```python
from build123d import *

# Parameters (mm, degrees)
SKIZZE1_R                       = 90
AUFSATZ_LINEAR_AUSTRAGEN1_DEPTH = 5
SKIZZE2_W                       = 6
SKIZZE2_H                       = 10
AUFSATZ_LINEAR_AUSTRAGEN2_DEPTH = 14
FASE1_SIZE                      = 14
SKIZZE3_R                       = 2.15
SCHNITT_LINEAR_AUSTRAGEN1_DEPTH = 42
KREISMUSTER1_COUNT              = 3
FASE1_OF_KREISMUSTER1_SIZE      = 14
AUFSATZ_LINEAR_AUSTRAGEN3_DEPTH = 3
AUFSATZ_LINEAR_AUSTRAGEN4_DEPTH = 3
SCHNITT_LINEAR_AUSTRAGEN2_REACH = 129.754
SKIZZE7_R                       = 1.75
KREISMUSTER2_COUNT              = 4
SCHNITT_LINEAR_AUSTRAGEN3_REACH = 130.69
SKIZZE8_R                       = 10
FASE2_SIZE                      = 0.5


with BuildPart() as part:
    # Skizze1 → Aufsatz-Linear austragen1 (new body)
    with BuildSketch(Plane(origin=(0, 0, 0), x_dir=(1, 0, 0), z_dir=(0, 1, 0))):
        with Locations(Location((0, 0, 0), (0, 0, 270))):
            Circle(SKIZZE1_R)
    extrude(amount=AUFSATZ_LINEAR_AUSTRAGEN1_DEPTH)

    # Skizze2 → Aufsatz-Linear austragen2 (add)
    with BuildSketch(Plane.XZ):
        with Locations((-18, 35)):
            Rectangle(SKIZZE2_W, SKIZZE2_H)
        with Locations((18, 35)):
            Rectangle(SKIZZE2_W, SKIZZE2_H)
    aufsatz_linear_austragen2 = extrude(amount=AUFSATZ_LINEAR_AUSTRAGEN2_DEPTH)

    # Fase1
    fase1_edges = [part.edges().sort_by_distance(p)[0] for p in [
        (18, 0, 40),
        (-18, 0, 40),
    ]]
    chamfer(fase1_edges, length=FASE1_SIZE - 0.0001)  # a hair under: the kernel refuses the full size

    # Skizze3 → Schnitt-Linear austragen1 (cut)
    with BuildSketch(Plane(origin=(21, 0, 0), x_dir=(0, 0, -1), z_dir=(1, 0, 0))):
        with Locations((-35, -7)):
            Circle(SKIZZE3_R)
    schnitt_linear_austragen1 = extrude(amount=-SCHNITT_LINEAR_AUSTRAGEN1_DEPTH, mode=Mode.SUBTRACT)

    # Kreismuster1: Aufsatz-Linear austragen2, Schnitt-Linear austragen1 ×3 about axis
    kreismuster1_axis = Axis((0, 0, 0), (0, 1, 0))
    add([aufsatz_linear_austragen2.rotate(kreismuster1_axis, i * 360 / KREISMUSTER1_COUNT) for i in range(1, KREISMUSTER1_COUNT)])
    add([schnitt_linear_austragen1.rotate(kreismuster1_axis, i * 360 / KREISMUSTER1_COUNT) for i in range(1, KREISMUSTER1_COUNT)], mode=Mode.SUBTRACT)

    # Fase1 of Kreismuster1
    fase1_of_kreismuster1_edges = [part.edges().sort_by_distance(p)[0] for p in [
        (25.641016151, 0, -35.588457268),
        (43.641016151, 0, -4.411542732),
        (-43.641016151, 0, -4.411542732),
        (-25.641016151, 0, -35.588457268),
    ]]
    chamfer(fase1_of_kreismuster1_edges, length=FASE1_OF_KREISMUSTER1_SIZE - 0.0001)  # a hair under: the kernel refuses the full size

    # Skizze4 → Aufsatz-Linear austragen3 (add)
    with BuildSketch(Plane.XZ):
        with BuildLine():
            ThreePointArc((-70.255477849, -23.241510972), (-64.08587988, 37), (-15, 72.463784058))
            Line((-15, 72.463784058), (-15, 78.581168228))
            ThreePointArc((-15, 78.581168228), (-69.282032303, 40), (-75.553287944, -26.300203057))
            Line((-75.553287944, -26.300203057), (-70.255477849, -23.241510972))
        make_face()
        with BuildLine():
            Line((15, 78.581168228), (15, 72.463784058))
            ThreePointArc((15, 72.463784058), (57.384666942, 46.722585545), (74, 0))
            ThreePointArc((74, 0), (73.057872132, -11.770612542), (70.255477849, -23.241510972))
            Line((70.255477849, -23.241510972), (75.553287944, -26.300203057))
            ThreePointArc((75.553287944, -26.300203057), (78.880488828, -13.336734317), (80, 0))
            ThreePointArc((80, 0), (61.64414003, 50.990195136), (15, 78.581168228))
        make_face()
        with BuildLine():
            ThreePointArc((55.255477849, -49.222273086), (0, -74), (-55.255477849, -49.222273086))
            Line((-55.255477849, -49.222273086), (-60.553287944, -52.280965171))
            ThreePointArc((-60.553287944, -52.280965171), (0, -80), (60.553287944, -52.280965171))
            Line((60.553287944, -52.280965171), (55.255477849, -49.222273086))
        make_face()
        with BuildLine():
            Line((15.480762114, -33.186533479), (18.480762114, -27.990381057))
            ThreePointArc((18.480762114, -27.990381057), (0, -33.541019662), (-18.480762114, -27.990381057))
            Line((-18.480762114, -27.990381057), (-15.480762114, -33.186533479))
            ThreePointArc((-15.480762114, -33.186533479), (0, -36.619666847), (15.480762114, -33.186533479))
        make_face()
        with BuildLine():
            ThreePointArc((-33.480762114, -2.009618943), (-29.047375097, 16.770509831), (-15, 30))
            Line((-15, 30), (-21, 30))
            ThreePointArc((-21, 30), (-31.713561768, 18.309833424), (-36.480762114, 3.186533479))
            Line((-36.480762114, 3.186533479), (-33.480762114, -2.009618943))
        make_face()
        with BuildLine():
            ThreePointArc((15, 30), (28.531695489, 17.633557569), (33.541019662, 0))
            ThreePointArc((33.541019662, 0), (33.525951891, -1.005261069), (33.480762114, -2.009618943))
            Line((33.480762114, -2.009618943), (36.480762114, 3.186533479))
            ThreePointArc((36.480762114, 3.186533479), (31.713561768, 18.309833424), (21, 30))
            Line((21, 30), (15, 30))
        make_face()
    extrude(amount=AUFSATZ_LINEAR_AUSTRAGEN3_DEPTH)

    # Skizze6 → Aufsatz-Linear austragen4 (add)
    with BuildSketch(Plane.XZ):
        with BuildLine():
            Line((-24.543328812, -76.142136894), (-25.319785948, -79.039914373))
            ThreePointArc((-25.319785948, -79.039914373), (-22.491358823, -83.938893859), (-17.592379337, -81.110466734))
            Line((-17.592379337, -81.110466734), (-16.815922202, -78.212689255))
            Line((-16.815922202, -78.212689255), (-24.543328812, -76.142136894))
        make_face()
        with BuildLine():
            Line((24.543328812, -76.142136894), (16.815922202, -78.212689255))
            Line((16.815922202, -78.212689255), (17.592379337, -81.110466734))
            ThreePointArc((17.592379337, -81.110466734), (22.491358823, -83.938893859), (25.319785948, -79.039914373))
            Line((25.319785948, -79.039914373), (24.543328812, -76.142136894))
        make_face()
    aufsatz_linear_austragen4 = extrude(amount=AUFSATZ_LINEAR_AUSTRAGEN4_DEPTH)

    # Skizze7 → Schnitt-Linear austragen2 (cut, up to next)
    with BuildSketch(Plane.XZ.offset(3), mode=Mode.PRIVATE) as schnitt_linear_austragen2_sk1:
        with Locations(Location((-21.456082643, -80.075190553, 0), (0, 0, 270))):
            Circle(SKIZZE7_R)
    schnitt_linear_austragen2_tool1 = extrude(schnitt_linear_austragen2_sk1.sketch, amount=-SCHNITT_LINEAR_AUSTRAGEN2_REACH, mode=Mode.PRIVATE) & part.part
    # Skizze7 → Schnitt-Linear austragen2 (cut, up to next)
    with BuildSketch(Plane.XZ.offset(3), mode=Mode.PRIVATE) as schnitt_linear_austragen2_sk2:
        with Locations(Location((21.456082643, -80.075190553, 0), (0, 0, 270))):
            Circle(SKIZZE7_R)
    schnitt_linear_austragen2_tool2 = extrude(schnitt_linear_austragen2_sk2.sketch, amount=-SCHNITT_LINEAR_AUSTRAGEN2_REACH, mode=Mode.PRIVATE) & part.part
    schnitt_linear_austragen2_1 = schnitt_linear_austragen2_tool1.solids().sort_by_distance((-21.456083, -3, -80.075191))[0]
    add(schnitt_linear_austragen2_1, mode=Mode.SUBTRACT)
    schnitt_linear_austragen2_2 = schnitt_linear_austragen2_tool2.solids().sort_by_distance((21.456083, -3, -80.075191))[0]
    add(schnitt_linear_austragen2_2, mode=Mode.SUBTRACT)
    schnitt_linear_austragen2 = schnitt_linear_austragen2_1 + schnitt_linear_austragen2_2  # Schnitt-Linear austragen2 as one shape, for the pattern or mirror that repeats it

    # Kreismuster2: Aufsatz-Linear austragen4, Schnitt-Linear austragen2 ×4 about axis
    kreismuster2_axis = Axis((0, 0, 0), (0, 1, 0))
    add([aufsatz_linear_austragen4.rotate(kreismuster2_axis, i * 360 / KREISMUSTER2_COUNT) for i in range(1, KREISMUSTER2_COUNT)])
    add([schnitt_linear_austragen2.rotate(kreismuster2_axis, i * 360 / KREISMUSTER2_COUNT) for i in range(1, KREISMUSTER2_COUNT)], mode=Mode.SUBTRACT)

    # Skizze8 → Schnitt-Linear austragen3 (cut, up to next)
    with BuildSketch(Plane(origin=(0, 5, 0), x_dir=(1, 0, 0), z_dir=(0, 1, 0)), mode=Mode.PRIVATE) as schnitt_linear_austragen3_sk1:
        with Locations(Location((0, 0, 0), (0, 0, 270))):
            Circle(SKIZZE8_R)
    schnitt_linear_austragen3_tool1 = extrude(schnitt_linear_austragen3_sk1.sketch, amount=-SCHNITT_LINEAR_AUSTRAGEN3_REACH, mode=Mode.PRIVATE) & part.part
    add(schnitt_linear_austragen3_tool1.solids().sort_by_distance((0, 5, 0))[0], mode=Mode.SUBTRACT)

    # Fase2
    fase2_edges = [part.edges().sort_by_distance(p)[0] for p in [
        (0, 5, -90),
    ]]
    chamfer(fase2_edges, length=FASE2_SIZE)


solid = part.part
```
Could you check a few things on this model? Use its own coordinates, in mm. A direction names the side the tool comes from. Round coordinates to 2 decimals unless told otherwise and drop trailing zeros. Loops run counter-clockwise (first coordinate to the right, second up) from the corner with the lowest first, then second, coordinate; pieces in that order, holes last.
Q1. For P1, Ø5.5, axis at x = 80.08, z = -21.46, coming from the -Y side; P2, Ø1.5, axis at y = -6, z = -11.5, coming from the +X side; P3, Ø11, axis at y = -9.5, z = 36.5, coming from the +X side, each with a flat end and sliding along its axis, tell me the tip position at first contact or that it passes through.
Q2. Thinking about a two-plate mould opening in Z: for faces 1 (the flat face through (0, -3, -76)), 2 (the flat face through (-44.418, -5.346, -1.396)), which applies, pulls with the +Z half, pulls with the -Z half, needs draft (parallel to the pull), parting line crosses it, or undercut?
Q3. I want a section at B-B (z = 35). Give the number of separate pieces and of enclosed holes in the cut face, and give its area (3 significant figures).
Q4. On a 3-axis mill with a long thin cutter (end or side, diameter ignored), from which of +Z, -Z, +X, -X, +Y, -Y can I reach the whole of each face in a straight line? I mean faces 3 (the flat face through (-15, -5, 39)), 4 (the flat face through (49.639, -7.098, -7.826)), 5 (the flat face through (18, -8, 30)), 6 (the flat face through (31.64, -7.1, -39)). Say none if no direction works.
Q5. I want a section at A-A (x = 0). Write out the boundary of the cut face in (y, z).
Q6. Please list where these lines run through material, in increasing order: L1, parallel to X at y = -6, z = 37; L2, parallel to Y at x = -19.6, z = 35; L3, parallel to Z at x = -49, y = -0.25.
Answer below:
1. P1: stops at y = -3
1. P2: stops at x = 49.75
1. P3: stops at x = 21
2. face 1: needs draft
2. face 2: undercut
3. separate pieces: 3
3. enclosed holes: 0
3. area: 986 mm2
4. face 3: +Z, -Y
4. face 4: -Y
4. face 5: +X, -X, -Y
4. face 6: +X, -Y
5. outline: (-3, -80) - (0, -80) - (0, -90) - (4.5, -90) - (5, -89.5) - (5, -10) - (0, -10) - (0, -33.54) - (-3, -33.54) - (-3, -36.62) - (0, -36.62) - (0, -74) - (-3, -74) - close; (0, 10) - (5, 10) - (5, 89.5) - (4.5, 90) - (0, 90) - close
6. L1: x = -21 to -15, 15 to 21
6. L2: y = -14 to -9.15, -4.85 to 5
6. L3: z = -63.24 to -55.45, -10.97 to -4.04, 55.45 to 63.24
